Source: CAD feature listing. Evaluate the final solid. Frame: model axes, mm. A direction names the side the tool comes from. Coordinates: 2 decimals unless noted, no trailing zeros. Order: outer loops, then holes, each group sorted by start corner. A loop starts at its lowest first (then second) coordinate and runs counter-clockwise, first axis right, second up. Notation, with made-up numbers: (74.25, -28.75) -> (84.25, -28.75) arc R23 cw to (84.25, 0.25) -> close; hole circle Ø7 at (58, 41). An arc over 180 degrees is marked (long way). Put each result on its own line as item: value.
Autodesk Inventor part; units mm, degrees
ref_plane "YZ Plane" through (0, 0, 0) normal (1, 0, 0) x (0, 1, 0)
ref_plane "XZ Plane" through (0, 0, 0) normal (0, 1, 0) x (-1, 0, 0)
ref_plane "XY Plane" through (0, 0, 0) normal (0, 0, 1) x (1, 0, 0)
sketch "Sketch1" plane through (0, 0, 0) normal (0, 0, 1) x (1, 0, 0)
  line L0 (0, 0) -> (861.06, 0)
  line L1 (861.06, 0) -> (861.06, 549.275)
  line L2 (861.06, 549.275) -> (0, 549.275)
  line L3 (0, 549.275) -> (0, 0)
  dimension "d2" = 861.06
  dimension "d3" = 549.275
extrude "Extrusion1" add sketch "Sketch1" along normal blind 4.7625
sketch "Sketch2" plane through (0, 0, 0) normal (0, 0, -1) x (-1, 0, 0)
  line L0 (-888.4793, 12.7) -> (25.9207, 12.7)
  line L1 (-12.1803, 12.7) -> (-12.1803, 536.575)
  line L2 (-850.3793, 12.7) -> (-850.3793, 536.575)
  line L3 (-888.4793, 536.575) -> (25.9207, 536.575)
  line L4 (-12.1803, 536.575) -> (-850.3793, 536.575)
  line L5 (-850.3793, 536.575) -> (-850.3793, 12.7)
  line L6 (-850.3793, 12.7) -> (-12.1803, 12.7)
  line L7 (-12.1803, 12.7) -> (-12.1803, 536.575)
  point P0 (0, 0)
extrude "Extrusion2" add sketch "Sketch2" along normal blind 25.4
properties part number "gatorboard_01875in"
1. Cut plane C-C on z = -5. Output: boundary loops of the cut face in (x, y) (3 decimals).
Numbers:
outline: (12.18, 12.7) -> (850.379, 12.7) -> (850.379, 536.575) -> (12.18, 536.575) -> close
2. First-contact query: pin 1 (1.5 mm diameter, centred on y = 97.5, z = -14, fed in from +X); pin 2 (1 mm diameter, centred on x = 575, z = -3.5, fed in from -Y); pin 3 (1 mm diameter, centred on x = 657, z = -2.5, fed in from +Y) (3 decimals). Flat tips, straight axial feed; report the tip coordinate or a pass-through.
Numbers:
pin 1: stops at x = 850.38
pin 2: stops at y = 12.7
pin 3: stops at y = 536.575
3. Pull-direction query (X, two-part tool) for faces 4 (the flat face through (850.379, 271, -13)), 5 (the flat face through (12.18, 271, -13)), 6 (the flat face through (425, 278, 4.762)); classes: pulls with the +X half, pulls with the -X half, needs draft (parallel to the pull), parting line crosses it, or undercut.
Numbers:
face 4: pulls with the +X half
face 5: pulls with the -X half
face 6: needs draft
4. Ray query, line 1 along Y through (x, z) = (738, -7) (3 decimals); line 2 along X through (y, z) = (276.5, -8.5). Return the intervals inside material, ascending.
Numbers:
line 1: y = 12.7 to 536.575
line 2: x = 12.18 to 850.38
5. Set-up query: faces 1 (the flat face through (437, 536.575, -13)), 2 (the flat face through (437, 278, -25.4)), 3 (the flat face through (437, 12.7, -13)). Return all of +Z, -Z, +X, -X, +Y, -Y with unobstructed straight access to the full face (end or side cutting, diameter ignored); none if empty.
Numbers:
face 1: -Z, +X, -X, +Y
face 2: -Z, +X, -X, +Y, -Y
face 3: -Z, +X, -X, -Y
6. Cut plane A-A on y = 38. Output: boundary loops of the cut face in (x, z).
Numbers:
outline: (0, 0) -> (12.18, 0) -> (12.18, -25.4) -> (850.38, -25.4) -> (850.38, 0) -> (861.06, 0) -> (861.06, 4.76) -> (0, 4.76) -> close
7. Cut plane B-B on x = 191. Output: boundary loops of the cut face in (y, z) (1 decimal), plus the area to 3 significant figures.
Numbers:
outline: (0, 0) -> (12.7, 0) -> (12.7, -25.4) -> (536.6, -25.4) -> (536.6, 0) -> (549.3, 0) -> (549.3, 4.8) -> (0, 4.8) -> close
area: 15,900 mm2
